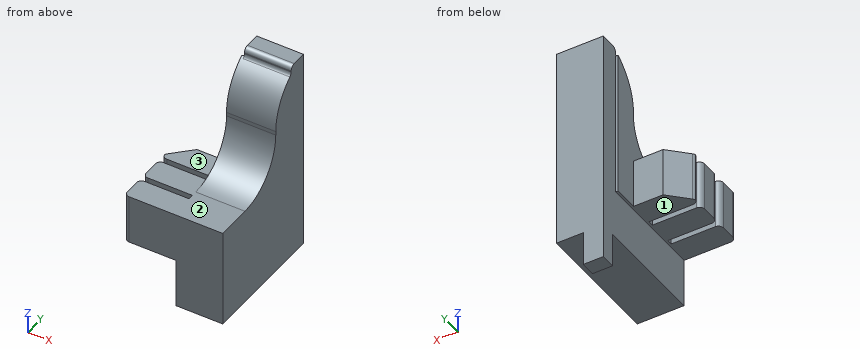
```python
from build123d import *

# Parameters (mm, degrees)
BOSS_EXTRU_1_DEPTH = 10
ESQUISSE2_W        = 9.5
ESQUISSE2_H        = 22.2
BOSS_EXTRU_2_DEPTH = 10
ESQUISSE3_W        = 10
ESQUISSE3_H        = 5
BOSS_EXTRU_3_DEPTH = 20
CONG_1_R           = 10
CHANFREIN1_SIZE    = 4
CONG_3_R           = 1
ESQUISSE5_W        = 9.5
ESQUISSE5_H        = 4.718482058
BOSS_EXTRU_5_DEPTH = 4
ESQUISSE6_W        = 4.048947881
ESQUISSE6_H        = 3
BOSS_EXTRU_6_DEPTH = 7
ESQUISSE7_W        = 9.5
ESQUISSE7_H        = 4
BOSS_EXTRU_7_DEPTH = 37
CONG_4_R           = 11
CONG_6_R           = 1


with BuildPart() as part:
    # Esquisse1 → Boss.-Extru.1 (new body)
    with BuildSketch(Plane.XY):
        Polygon((0, 0), (10, 0), (10, -22.2), (-10, -22.2), (-10, -17.2), (0, -17.2), (0, -16.1), (-10, -16.1), (-10, -11.1), (0, -11.1), (0, -10), (-10, -10), (-10, -5), (0, -5), align=None)
    extrude(amount=BOSS_EXTRU_1_DEPTH)

    # Esquisse2 → Boss.-Extru.2 (add)
    with BuildSketch(Plane(origin=(0, 0, 0), x_dir=(-1, 0, 0), z_dir=(0, 0, -1))):
        with Locations((-5.25, -11.1)):
            Rectangle(ESQUISSE2_W, ESQUISSE2_H)
    extrude(amount=BOSS_EXTRU_2_DEPTH)

    # Esquisse3 → Boss.-Extru.3 (add)
    with BuildSketch(Plane.XY.offset(10)):
        with Locations((5, -2.5)):
            Rectangle(ESQUISSE3_W, ESQUISSE3_H)
    extrude(amount=BOSS_EXTRU_3_DEPTH)

    # Congé1
    # the kernel refuses this fillet: 10 mm, written as the material it adds along each edge
    with BuildSketch(Plane(origin=(0, -5, 10), x_dir=(0, -1, 0), z_dir=(1, 0, 0))) as cong_1_piece_1:
        with BuildLine():
            CenterArc((CONG_1_R, -CONG_1_R), CONG_1_R, 90, 90)
            Line((0, -CONG_1_R), (0, 0))
            Line((0, 0), (CONG_1_R, 0))
        make_face()
    extrude(amount=10)

    # Chanfrein1
    chanfrein1_edges = [part.edges().sort_by_distance(p)[0] for p in [
        (-10, -5, 5),
    ]]
    chamfer(chanfrein1_edges, length=CHANFREIN1_SIZE)

    # Congé3
    # the kernel refuses this fillet: 1 mm, written as the material it takes off along each edge
    with BuildSketch(Plane(origin=(-10, -22.2, -2.5), x_dir=(1, 0, 0), z_dir=(0, 0, 1)), Plane(origin=(-10, -17.2, -2.5), x_dir=(0, -1, 0), z_dir=(0, 0, 1))) as cong_3_piece_1:
        with BuildLine():
            CenterArc((CONG_3_R, CONG_3_R), CONG_3_R, 180, 90)
            Line((0, CONG_3_R), (0, 0))
            Line((0, 0), (CONG_3_R, 0))
        make_face()
    extrude(amount=15, mode=Mode.SUBTRACT)
    with BuildSketch(Plane(origin=(-10, -16.1, -2.5), x_dir=(0, 1, 0), z_dir=(0, 0, 1)), Plane(origin=(-10, -11.1, -2.5), x_dir=(1, 0, 0), z_dir=(0, 0, 1)), Plane(origin=(-10, -10, -2.5), x_dir=(0, 1, 0), z_dir=(0, 0, 1))) as cong_3_piece_2:
        with BuildLine():
            CenterArc((CONG_3_R, -CONG_3_R), CONG_3_R, 90, 90)
            Line((0, -CONG_3_R), (0, 0))
            Line((0, 0), (CONG_3_R, 0))
        make_face()
    extrude(amount=15, mode=Mode.SUBTRACT)
    with BuildSketch(Plane(origin=(-10, -9, -1.035533906), x_dir=(0, -1, 0), z_dir=(0, 0, 1))) as cong_3_piece_3:
        with BuildLine():
            CenterArc((CONG_3_R * 0.414213562373, CONG_3_R), CONG_3_R, 225, 45)
            Line((-CONG_3_R * 0.292893218813, CONG_3_R * 0.292893218813), (0, 0))
            Line((0, 0), (CONG_3_R * 0.414213562373, 0))
        make_face()
    extrude(amount=12.071067812, mode=Mode.SUBTRACT)

    # Esquisse5 → Boss.-Extru.5 (add)
    with BuildSketch(Plane(origin=(0, 0, 0), x_dir=(1, 0, 0), z_dir=(0, 1, 0))):
        with Locations((5.25, 7.640758971)):
            Rectangle(ESQUISSE5_W, ESQUISSE5_H)
    extrude(amount=BOSS_EXTRU_5_DEPTH)

    # Esquisse6 → Boss.-Extru.6 (add)
    with BuildSketch(Plane(origin=(0, 0, -10), x_dir=(-1, 0, 0), z_dir=(0, 0, -1))):
        with Locations((-2.524473941, 2.5)):
            Rectangle(ESQUISSE6_W, ESQUISSE6_H)
    extrude(amount=BOSS_EXTRU_6_DEPTH)

    # Esquisse7 → Boss.-Extru.7 (add)
    with BuildSketch(Plane.XY.offset(-5.281517942)):
        with Locations((5.25, 2)):
            Rectangle(ESQUISSE7_W, ESQUISSE7_H)
    extrude(amount=BOSS_EXTRU_7_DEPTH)

    # Congé4
    # the kernel refuses this fillet: 11 mm, written as the material it takes off along each edge
    with BuildSketch(Plane(origin=(-23.048861143, -5, 30), x_dir=(0, 1.0, -1.1723955140032709e-12), z_dir=(1, 0, 0))) as cong_4_piece_1:
        with BuildLine():
            CenterArc((11, -9.219544457), CONG_4_R, 123.055731151, 56.944268849)
            Line((0, -9.219544457), (-0.22, -9.219544457))
            Line((-0.22, -9.219544457), (-0.22, 0))
            Line((-0.22, 0), (0, 0.22))
            ThreePointArc((0, 0.22), (2.5, 0.22), (4.88, 0.184390889))
            Line((4.88, 0.184390889), (5, 0))
        make_face()
    extrude(amount=56.097722287, mode=Mode.SUBTRACT)

    # Congé6
    cong_6_edges = [part.edges().sort_by_distance(p)[0] for p in [
        (5.25, 0, 31.718482058),
        (5.25, 0, 30),
    ]]
    fillet(cong_6_edges, radius=CONG_6_R)


solid = part.part
```
For this review, take the finished solid that the model builds, in its own axes (mm). Face numbers are marked on the shaded views. A direction names the side the tool comes from. Give positions to 0.01 mm unless a question says otherwise; leave off trailing zeros. Write each loop counter-clockwise with the first axis right and the second up, starting at its lowest first coordinate (ties: lowest second). Pieces come first, ordered by that corner, then holes. Notation, with made-up numbers: M 35,-11.75 L 46,-11.75 A23 ccw 46,22.25 Z; hole C -21,34.5 d1. An arc over 180 degrees is marked long. One line per item, written item: value.
1) For line 1 (Y direction, x = -9, z = 2); line 2 (Y direction, x = -8.25, z = 4.5); line 3 (X direction, y = -18.25, z = -3), list the stretches that pass through material, from the lowest coordinate up. Write a range as from..to.
Results are:
line 1: y = -22.2..-17.2, -16.1..-11.1, -10..-8
line 2: y = -22.2..-17.2, -16.1..-11.1, -10..-7.25
line 3: x = 0.5..10
2) For the marked faces 1, 2 and 3, list the 3-axis set-ups (+Z, -Z, +X, -X, +Y, -Y) from which the entire face can be reached by the end or side of a thin tool; tool diameter is ignored.
Results are:
face 1: -Z, -X, +Y, -Y
face 2: +Z, -X, -Y
face 3: +Z, -X, +Y, -Y
3) Take a section at B-B, the plane z = 3. Write out the cut boundary in (x, y), then the cut area to 3 significant figures.
Results are:
outline: M -10,-21.2 A1 ccw -9,-22.2 L 10,-22.2 L 10,4 L 0.5,4 L 0.5,0 L 0,0 L 0,-5 L -6,-5 L -9.71,-8.71 A1 ccw -9.98,-9.21 A1 ccw -9,-10 L 0,-10 L 0,-11.1 L -9,-11.1 A1 ccw -10,-12.1 L -10,-15.1 A1 ccw -9,-16.1 L 0,-16.1 L 0,-17.2 L -9,-17.2 A1 ccw -10,-18.2 Z
area: 401 mm²
4) For P1, Ø2, axis at x = 6, y = -16.5, coming from the -Z side; P2, Ø3.5, axis at x = -0.5, y = -14.5, coming from the +Z side; P3, Ø1.2, axis at x = 3, z = -12.5, coming from the -Y side; P4, Ø6, axis at x = -1, z = -11.5, coming from the -Y side, all flat-tipped, find the tip position at first contact; note any pin that passes through.
Results are:
P1: stops at z = -10
P2: stops at z = 10.24
P3: stops at y = 1
P4: stops at y = -22.2
5) Take a section at C-C, the plane x = -7.25. Write out the cut boundary in (y, z), then the cut area to 4 significant figures.
Results are:
outline: M -22.2,0 L -17.2,0 L -17.2,10 L -22.2,10 Z; M -16.1,0 L -11.1,0 L -11.1,10 L -16.1,10 Z; M -10,0 L -6.25,0 L -6.25,10 L -10,10 Z
area: 137.5 mm²
6) Take a section at D-D, the plane y = -20.5. Write out the cut boundary in (x, z), then the cut area to 3 significant figures.
Results are:
outline: M -10,0 L 0.5,0 L 0.5,-10 L 10,-10 L 10,10 L -10,10 Z
area: 295 mm²
7) Take a section at A-A, the plane x = -1.5. Write out the cut boundary in (y, z).
Results are:
outline: M -22.2,0 L -17.2,0 L -17.2,10 L -22.2,10 Z; M -16.1,0 L -11.1,0 L -11.1,10 L -16.1,10 Z; M -10,0 L -5,0 L -5,10 L -10,10 Z
